```python
from build123d import *

# Parameters (mm, degrees)
SKETCH1_R           = 1.5
BOSS_EXTRUDE1_DEPTH = 7
SKETCH2_R           = 2.5
BOSS_EXTRUDE2_DEPTH = 0.5
SKETCH3_R           = 1.5
BOSS_EXTRUDE3_DEPTH = 17
CHAMFER1_SIZE       = 1
CHAMFER1_SIZE2      = 1.732050808


with BuildPart() as part:
    # Sketch1 → Boss-Extrude1 (new body)
    with BuildSketch(Plane(origin=(0, 0, 0), x_dir=(1, 0, 0), z_dir=(0, 1, 0))):
        with Locations(Location((0, 0, 0), (0, 0, 270))):
            Circle(SKETCH1_R)
    extrude(amount=BOSS_EXTRUDE1_DEPTH)

    # Sketch2 → Boss-Extrude2 (add)
    with BuildSketch(Plane(origin=(0, 7, 0), x_dir=(1, 0, 0), z_dir=(0, 1, 0))):
        with Locations(Location((0, 0, 0), (0, 0, 270))):
            Circle(SKETCH2_R)
    extrude(amount=BOSS_EXTRUDE2_DEPTH)

    # Sketch3 → Boss-Extrude3 (add)
    with BuildSketch(Plane(origin=(0, 7.5, 0), x_dir=(1, 0, 0), z_dir=(0, 1, 0))):
        with Locations(Location((0, 0, 0), (0, 0, 270))):
            Circle(SKETCH3_R)
    extrude(amount=BOSS_EXTRUDE3_DEPTH)

    # Chamfer1
    chamfer1_edges = [part.edges().sort_by_distance(p)[0] for p in [
        (0, 24.5, -1.5),
    ]]
    chamfer1_side = [part.faces().sort_by_distance(p)[0] for p in [
        (0, 24.5, 0),
    ]]
    chamfer(chamfer1_edges, length=CHAMFER1_SIZE, length2=CHAMFER1_SIZE2, reference=chamfer1_side[0])


solid = part.part
```
Geometry: final body of the model. Coordinates: model frame, mm. A direction names the side the tool comes from. Coordinates: 2 decimals unless noted, no trailing zeros. Order: outer loops, then holes, each group sorted by start corner. A loop starts at its lowest first (then second) coordinate and runs counter-clockwise, first axis right, second up. Notation, with made-up numbers: (72, 2.25) - (106, 2.25) arc R18 cw to (106, 20.25) - close; hole circle Ø6 at (15.25, -20.5). An arc over 180 degrees is marked (long way). Write each question's results on one line, items separated by ' | '.
1) Section D-D, the plane x = 2. Return loops of the section in (y, z), plus the area to 3 significant figures.
Results list:
outline: (7, -1.5) - (7.5, -1.5) - (7.5, 1.5) - (7, 1.5) - close | area: 1.50 mm^2
2) Section A-A, the plane x = 0. Return loops of the section in (y, z).
Results list:
outline: (0, -1.5) - (7, -1.5) - (7, -2.5) - (7.5, -2.5) - (7.5, -1.5) - (22.77, -1.5) - (24.5, -0.5) - (24.5, 0.5) - (22.77, 1.5) - (7.5, 1.5) - (7.5, 2.5) - (7, 2.5) - (7, 1.5) - (0, 1.5) - close
3) Set-up query: faces 1 (the flat face through (-2, 7.5, 0)), 2 (the cylindrical face through (-2.44, 7.25, -0.54)), 3 (the cylindrical face through (0.45, 3.45, 1.43)). Return all of +Z, -Z, +X, -X, +Y, -Y with unobstructed straight access to the full face (end or side cutting, diameter ignored); none if empty.
Results list:
face 1: +Y | face 2: +Y, -Y | face 3: -Y
4) Section C-C, the plane y = 10. Return loops of the section in (x, z).
Results list:
outline: circle Ø3 at (0, 0)
5) Line query: line 1 (X direction, y = 14.75, z = 0); line 2 (Y direction, x = 1.65, z = -0.65); line 3 (X direction, y = 8, z = 1). Output: solid intervals per line, ascending. Write a range as from..to.
Results list:
line 1: -1.5..1.5 | line 2: 7..7.5 | line 3: -1.12..1.12
6) Section B-B, the plane z = 0. Return loops of the section in (x, y).
Results list:
outline: (-2.5, 7) - (-1.5, 7) - (-1.5, 0) - (1.5, 0) - (1.5, 7) - (2.5, 7) - (2.5, 7.5) - (1.5, 7.5) - (1.5, 22.77) - (0.5, 24.5) - (-0.5, 24.5) - (-1.5, 22.77) - (-1.5, 7.5) - (-2.5, 7.5) - close
7) Pin query (flat end, axial travel): pin 1 (1.5 mm diameter, centred on x = 0, y = 3, fed in from -Z); pin 2 (3 mm diameter, centred on x = 0, y = 21, fed in from +Z). Return the tip coordinate at first contact, or that it passes through.
Results list:
pin 1: z = -1.5 | pin 2: z = 1.5
